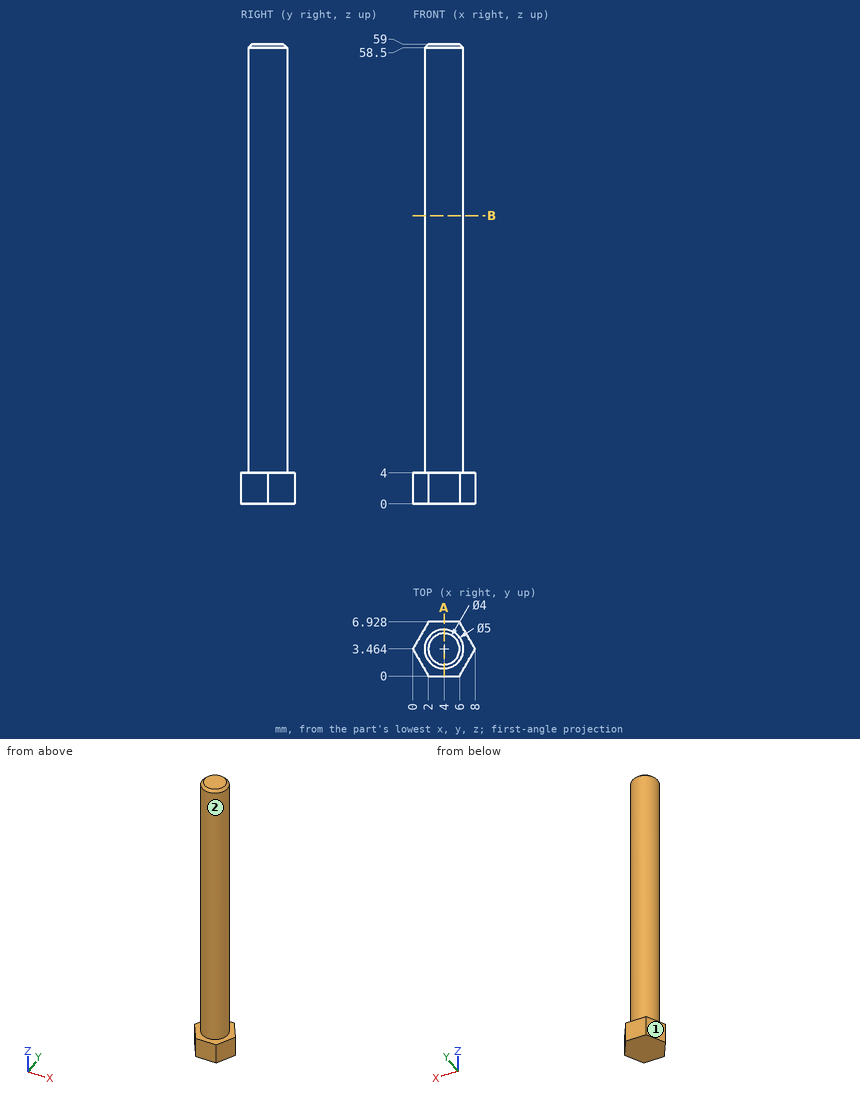
Here's the drawing with two shaded views (mm, measured from the low corner). I have some questions. A direction names the side the tool comes from. Round coordinates to 2 decimals unless told otherwise and drop trailing zeros. Loops run counter-clockwise (first coordinate to the right, second up) from the corner with the lowest first, then second, coordinate; pieces in that order, holes last. Notation, with made-up numbers: (36.25, 17) - (72.25, 17) arc R25 cw to (72.25, 56) - close; hole circle Ø3 at (70, -18). An arc over 180 degrees is marked (long way). Use CSV: the item, a comma, the result in double quotes.
Item 1: I need wall thicknesses on L1, parallel to Z at x = 5.75, y = 6; L2, parallel to Y at x = 5.5, z = 41 (1 decimal); L3, parallel to X at y = 5.75, z = 22. Which ranges of each line are inside material? Lowest first, please. Write a range as [from, to].
Here are the results:
L1,"z = [0, 4]"
L2,"y = [1.5, 5.5]"
L3,"x = [2.99, 5.01]"
Item 2: For the marked faces 1 and 2, which set-ups out of +Z, -Z, +X, -X, +Y, -Y let a thin tool reach every point of the face, with its end or its side?
Here are the results:
face 1,"+Z, -Z, -X, +Y"
face 2,"+Z"
Item 3: If we section it at A-A on x = 4: List the corners of the cut face in (y, z) for me.
Here are the results:
outline,"(0, 0) - (6.93, 0) - (6.93, 4) - (5.96, 4) - (5.96, 58.5) - (5.46, 59) - (1.46, 59) - (0.96, 58.5) - (0.96, 4) - (0, 4) - close"
Item 4: Will these pins go through, and if not, where does the flat tip stop? pin 1 (1 mm diameter, centred on x = 2.5, y = 1, fed in from +Z) (1 decimal); pin 2 (1.5 mm diameter, centred on y = 4, z = 47.5, fed in from +X).
Here are the results:
pin 1,"stops at z = 58.6"
pin 2,"stops at x = 6.5"
Item 5: If we section it at B-B on z = 37: List the corners of the cut face in (x, y) for me.
Here are the results:
outline,"circle Ø5 at (4, 3.46)"
